CAD build for the part. Positions are in the model's coordinates, mm. A direction names the side the tool comes from. Give positions to 0.01 mm unless a question says otherwise; leave off trailing zeros. Loops run counter-clockwise (first coordinate to the right, second up) from the corner with the lowest first, then second, coordinate; pieces in that order, holes last. Notation, with made-up numbers: (-34, -27) -> (17, -27) arc R9 ccw to (17, -20) -> close; hole circle Ø3 at (7.25, 77). An arc over 180 degrees is marked (long way). Use one line per item in the form item = value.
```python
from build123d import *

# Parameters (mm, degrees)
SKETCH1_W           = 120
SKETCH1_H           = 10
SKETCH1_R           = 1.9
BOSS_EXTRUDE1_DEPTH = 4
SKETCH2_R           = 1.95
CUT_EXTRUDE1_DEPTH  = 8
CHAMFER1_SIZE       = 0.5


with BuildPart() as part:
    # Sketch1 → Boss-Extrude1 (new, symmetric)
    with BuildSketch(Plane(origin=(0, 0, 0), x_dir=(1, 0, 0), z_dir=(0, 1, 0))):
        Rectangle(SKETCH1_W, SKETCH1_H)
        with Locations(Location((-50, 0, 0), (0, 0, 270))):
            Circle(SKETCH1_R, mode=Mode.SUBTRACT)
        with Locations(Location((50, 0, 0), (0, 0, 90))):
            Circle(SKETCH1_R, mode=Mode.SUBTRACT)
        with Locations(Location((0, 0, 0), (0, 0, 270))):
            Circle(SKETCH1_R, mode=Mode.SUBTRACT)
    extrude(amount=BOSS_EXTRUDE1_DEPTH, both=True)

    # Sketch2 → Cut-Extrude1 (cut)
    with BuildSketch(Plane.ZY.offset(60)):
        Circle(SKETCH2_R)
    cut_extrude1 = extrude(amount=-CUT_EXTRUDE1_DEPTH, mode=Mode.SUBTRACT)

    # Mirror1: Cut-Extrude1 across plane
    add(cut_extrude1.mirror(Plane(origin=(0, 0, 0), x_dir=(0, 0, 1), z_dir=(1, 0, 0))), mode=Mode.SUBTRACT)

    # Chamfer1
    chamfer1_edges = [part.edges().sort_by_distance(p)[0] for p in [
        (-50, -4, -1.9),
        (-50, 4, -1.9),
        (-60, 4, 0),
        (50, -4, 1.9),
        (50, 4, 1.9),
        (0, 4, 5),
        (0, -4, -1.9),
        (0, 4, -1.9),
        (-60, 0, -1.95),
        (60, 0, -1.95),
        (60, 4, 0),
        (0, -4, 5),
        (-60, -4, 0),
        (0, -4, -5),
        (60, -4, 0),
        (60, 0, 5),
        (-60, 0, 5),
        (-60, 0, -5),
        (60, 0, -5),
        (0, 4, -5),
    ]]
    chamfer(chamfer1_edges, length=CHAMFER1_SIZE)


solid = part.part
```
1. Cut at B-B, the plane y = 0. Write the cut outline in (x, z), then the cut area to 3 significant figures.
Result sheet:
outline = (-60, -4.5) -> (-59.5, -5) -> (59.5, -5) -> (60, -4.5) -> (60, -2.45) -> (59.5, -1.95) -> (52, -1.95) -> (52, 1.95) -> (59.5, 1.95) -> (60, 2.45) -> (60, 4.5) -> (59.5, 5) -> (-59.5, 5) -> (-60, 4.5) -> (-60, 2.45) -> (-59.5, 1.95) -> (-52, 1.95) -> (-52, -1.95) -> (-59.5, -1.95) -> (-60, -2.45) -> close; hole circle Ø3.8 at (-50, 0); hole circle Ø3.8 at (0, 0); hole circle Ø3.8 at (50, 0)
area = 1,100 mm^2
2. Cut at C-C, the plane z = 0. State how many separate pieces and enclosed holes the cut face has, then the cut area to 3 significant figures.
Result sheet:
separate_pieces = 4
enclosed_holes = 0
area = 804 mm^2
3. Tool access for faces 1 (the flat face through (-52, 0, -0.5)), 2 (the cylindrical face through (55.802, 1.318, -1.437)), 3 (the flat face through (-1, -4, 3)): list every direction of +Z, -Z, +X, -X, +Y, -Y with a clear straight run to the whole face (end or side of a thin tool).
Result sheet:
face_1 = -X
face_2 = +X
face_3 = +Z, -Z, +X, -X, -Y
4. Mould opens along Y. For faces 4 (the flat face through (-60, -2, 2)), 5 (the flat face through (-1, 4, 3)), 6 (the flat face through (52, 0, -0.5)) say: pulls with the +Y half, pulls with the -Y half, needs draft (parallel to the pull), parting line crosses it, or undercut.
Result sheet:
face_4 = needs draft
face_5 = pulls with the +Y half
face_6 = undercut
5. Cut at A-A, the plane x = 0. Write the cut outline in (y, z).
Result sheet:
outline = (-4, -4.5) -> (-3.5, -5) -> (3.5, -5) -> (4, -4.5) -> (4, -2.4) -> (3.5, -1.9) -> (-3.5, -1.9) -> (-4, -2.4) -> close; (-4, 2.4) -> (-3.5, 1.9) -> (3.5, 1.9) -> (4, 2.4) -> (4, 4.5) -> (3.5, 5) -> (-3.5, 5) -> (-4, 4.5) -> close
6. Drop flat-ended pins along their axis: P1, Ø3, axis at y = 0, z = 0, coming from the +X side; P2, Ø3, axis at x = 0, z = 0, coming from the +Y side; P3, Ø1.2, axis at y = -0.5, z = -0.5, coming from the -X side. Give the stop position or say it passes through.
Result sheet:
P1 = 52
P2 = through
P3 = -52
7. Drill centre lines: line 1 (Y direction, x = -56.75, z = 0); line 2 (X direction, y = 2, z = -1); line 3 (Z direction, x = 50, y = -0.25). Where is each one in solid material? Low to high.
Result sheet:
line_1 = -4 to -1.95, 1.95 to 4
line_2 = -59.79 to -51.62, -48.38 to -1.62, 1.62 to 48.38, 51.62 to 59.79
line_3 = -5 to -1.9, 1.9 to 5
